Can you work these out from the drawing? Everything is in mm from the part's minimum corner. A direction names the side the tool comes from. Coordinates: 2 decimals unless noted, no trailing zeros. Order: outer loops, then holes, each group sorted by start corner. A loop starts at its lowest first (then second) coordinate and runs counter-clockwise, first axis right, second up. Notation, with made-up numbers: (40, -34) -> (61, -34) arc R21 cw to (61, -13) -> close; hole circle Ø4 at (-35, 17). An arc over 180 degrees is marked (long way). Use a Markdown table: item, result. Add a question column.
1) If we section it at A-A (z = 11.43): Write out the boundary of the cut face in (x, y), plus the area to 3 significant figures.
2) If I drill on L1, parallel to X at y = 2.75, z = 11.43; L2, parallel to X at y = 2.5, z = 3.5; L3, parallel to X at y = 3, z = 18.5, over which ranges is the centre line in solid material (lowest first)? Write a range as [from, to].
3) Thinking about a two-plate mould opening in X: for the marked faces 3, 4 and 5, which applies, +X half, -X half, draft (parallel to the pull), parting line (faces both ways), or undercut?
4) Will these pins go through, and if not, where does the flat tip stop? pin 1 Ø2.5 at (x, z) = (20.93, 11.43) entering from +Y; pin 2 Ø3 at (x, z) = (13.5, 13) entering from +Y; pin 3 Ø1 at (x, y) = (4.5, 1) entering from +Z; pin 4 Ø2 at (x, y) = (15, 5) entering from +Z.
5) Which directions (+Z, -Z, +X, -X, +Y, -Y) give clear straight access to the entire face, cutting with the end or side of a thin tool? Please do the marked faces 1 and 2.
6) If we section it at B-B (y = 1.25): Write out the boundary of the cut face in (x, z).
7) If we section it at C-C (x = 20.93): Write out the boundary of the cut face in (y, z).
8) If we section it at D-D (x = 11.75): Write out the boundary of the cut face in (y, z), plus the area to 3 significant figures.
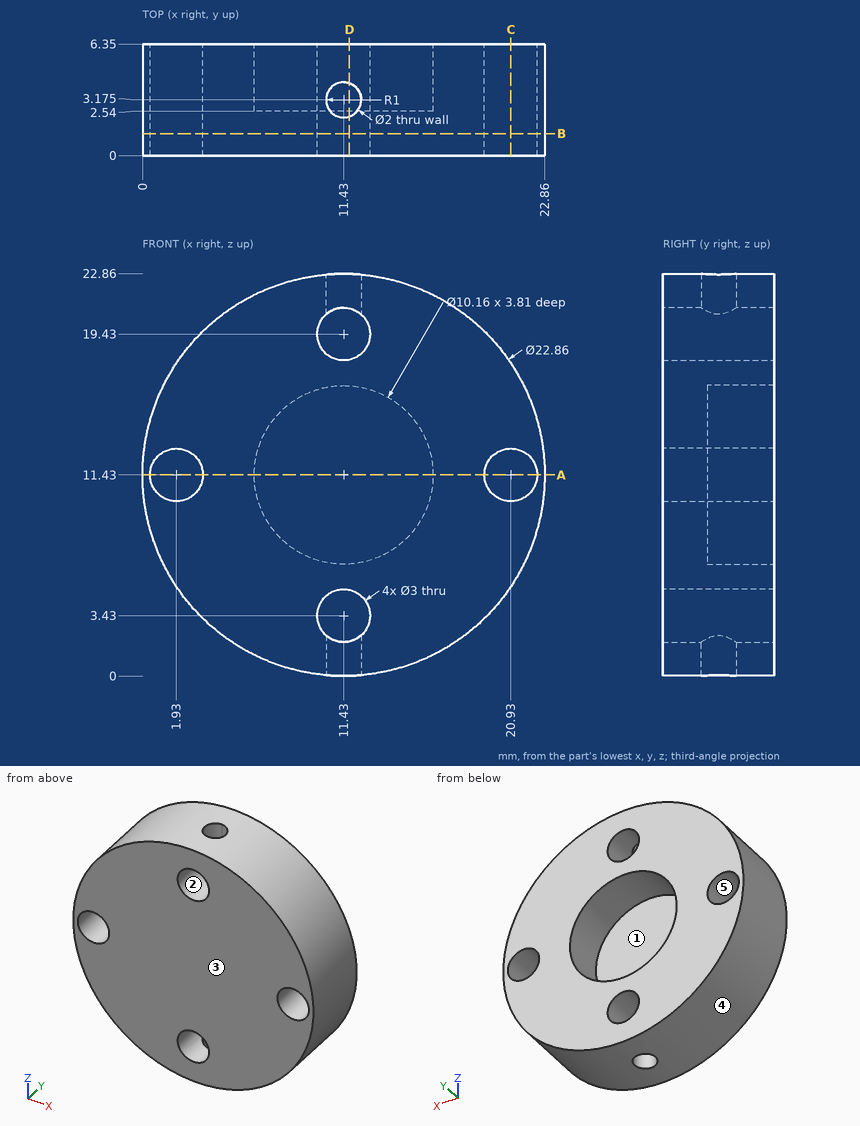
Answer sheet:
| question | item | result |
|---|---|---|
| 1 | outline | (0, 0) -> (0.43, 0) -> (0.43, 6.35) -> (0, 6.35) -> close; (3.43, 0) -> (19.43, 0) -> (19.43, 6.35) -> (16.51, 6.35) -> (16.51, 2.54) -> (6.35, 2.54) -> (6.35, 6.35) -> (3.43, 6.35) -> close; (22.43, 0) -> (22.86, 0) -> (22.86, 6.35) -> (22.43, 6.35) -> close |
| 1 | area | 68.4 mm2 |
| 2 | L1 | [0, 0.43], [3.43, 6.35], [16.51, 19.43], [22.43, 22.86] |
| 2 | L2 | [3.2, 9.93], [12.93, 19.66] |
| 2 | L3 | [2.45, 10.25], [12.61, 20.41] |
| 3 | face 3 | draft |
| 3 | face 4 | parting line |
| 3 | face 5 | undercut |
| 4 | pin 1 | through |
| 4 | pin 2 | y = 2.54 |
| 4 | pin 3 | z = 20.88 |
| 4 | pin 4 | z = 22.57 |
| 5 | face 1 | +Y |
| 5 | face 2 | +Y, -Y |
| 6 | outline | circle Ø22.86 at (11.43, 11.43); hole circle Ø3 at (1.93, 11.43); hole circle Ø3 at (11.43, 3.43); hole circle Ø3 at (11.43, 19.43); hole circle Ø3 at (20.93, 11.43) |
| 7 | outline | (0, 5.07) -> (6.35, 5.07) -> (6.35, 9.93) -> (0, 9.93) -> close; (0, 12.93) -> (6.35, 12.93) -> (6.35, 17.79) -> (0, 17.79) -> close |
| 8 | outline | (0, 0) -> (2.23, 0) -> (2.23, 1.96) -> (0, 1.96) -> close; (0, 4.9) -> (6.35, 4.9) -> (6.35, 6.36) -> (2.54, 6.36) -> (2.54, 16.5) -> (6.35, 16.5) -> (6.35, 17.96) -> (0, 17.96) -> close; (0, 20.9) -> (2.23, 20.9) -> (2.23, 22.86) -> (0, 22.86) -> close; (4.12, 0) -> (6.35, 0) -> (6.35, 1.96) -> (4.12, 1.96) -> close; (4.12, 20.9) -> (6.35, 20.9) -> (6.35, 22.86) -> (4.12, 22.86) -> close |
| 8 | area | 61.8 mm2 |
